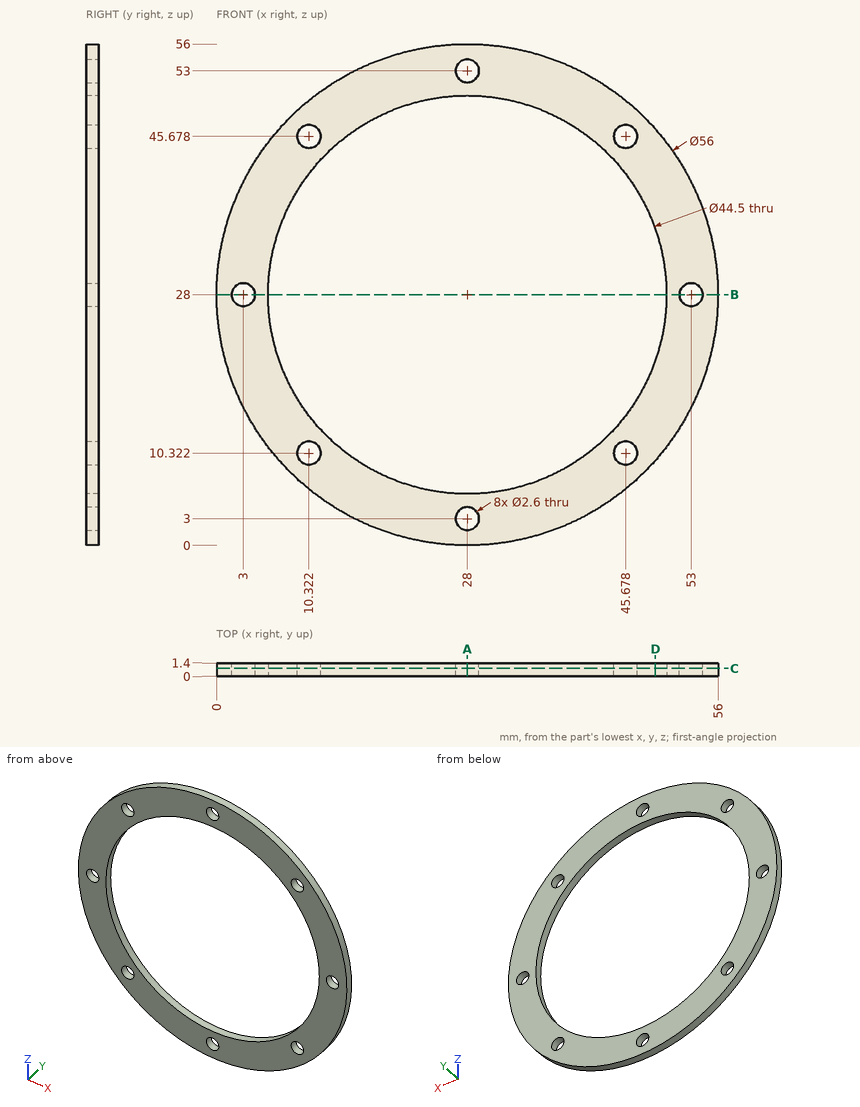
Source: three-view drawing plus pictorial views. Frame: mm from the lowest corner of the part. Round coordinates to 2 decimals unless told otherwise and drop trailing zeros. Loops run counter-clockwise (first coordinate to the right, second up) from the corner with the lowest first, then second, coordinate; pieces in that order, holes last. Notation, with made-up numbers: (0, -4.75) - (16, -4.75) arc R20 cw to (16, 12.25) - close; hole circle Ø11 at (6.5, 59). An arc over 180 degrees is marked (long way). Write each question's results on one line, items separated by ' | '. Start each with the question number.
1) Cut plane C-C on y = 0.85. Count the separate pieces of the cut face and the enclosed holes in it.
2) Line query: probe 1 along X at (y, z) = (1.25, 27); probe 2 along X at (y, z) = (0.7, 28.5) (1 decimal); probe 3 along Z at (x, y) = (24.5, 0.8). Output: solid intervals per line, ascending. Write a range as [from, to].
3) Cut plane B-B on z = 28. Return loops of the section in (x, y).
4) Cut plane D-D on x = 49. Return loops of the section in (y, z).
5) Cut plane A-A on x = 28. Return loops of the section in (y, z).
Verdict:
1) separate pieces: 1 | enclosed holes: 9
2) probe 1: x = [0.02, 2.17], [3.83, 5.77], [50.23, 52.17], [53.83, 55.98] | probe 2: x = [0, 1.8], [4.2, 5.8], [50.2, 51.8], [54.2, 56] | probe 3: z = [0.22, 6.03], [49.97, 55.78]
3) outline: (0, 0) - (1.7, 0) - (1.7, 1.4) - (0, 1.4) - close; (4.3, 0) - (5.75, 0) - (5.75, 1.4) - (4.3, 1.4) - close; (50.25, 0) - (51.7, 0) - (51.7, 1.4) - (50.25, 1.4) - close; (54.3, 0) - (56, 0) - (56, 1.4) - (54.3, 1.4) - close
4) outline: (0, 9.48) - (1.4, 9.48) - (1.4, 20.65) - (0, 20.65) - close; (0, 35.35) - (1.4, 35.35) - (1.4, 46.52) - (0, 46.52) - close
5) outline: (0, 0) - (1.4, 0) - (1.4, 1.7) - (0, 1.7) - close; (0, 4.3) - (1.4, 4.3) - (1.4, 5.75) - (0, 5.75) - close; (0, 50.25) - (1.4, 50.25) - (1.4, 51.7) - (0, 51.7) - close; (0, 54.3) - (1.4, 54.3) - (1.4, 56) - (0, 56) - close
